For this review, take the finished solid that the model builds, in its own axes (mm). A direction names the side the tool comes from. Give positions to 0.01 mm unless a question says otherwise; leave off trailing zeros. Order: outer loops, then holes, each group sorted by start corner. A loop starts at its lowest first (then second) coordinate and runs counter-clockwise, first axis right, second up. Notation, with made-up numbers: (4, 35) - (32, 35) arc R11 ccw to (32, 42) - close; hole circle Ø6 at (27, 61). An arc over 180 degrees is marked (long way). Use a Markdown table: item, result. Add a question column.
1) We need section C-C on z = 32. Write out the cut boundary in (x, y).
2) Wall thickness on L1, parallel to Z at x = 15.5, y = -8.5; L2, parallel to Y at x = -6, z = 14.5; L3, parallel to Z at x = -15.5, y = -6.25: over which ranges is each line inside the solid? List them lowest first.
3) Machinability: for faces 5 (the face through (-17, -9, 10)), 6 (the face through (17, 0, 35)), 7 (the face through (0, -17, 5)), which of the approach directions +Z, -Z, +X, -X, +Y, -Y give a long, thin tool a straight path to every point of the face, cutting with its end or side? Answer none if there is none.
4) We need section D-D on y = -7.5. Write out the cut boundary in (x, z).
5) Mouldability with a two-part tool opening along Z and no side actions: class faces 1 (the face through (17, -9, 10)), 2 (the face through (20, -16, 20)), 3 (the face through (0, -16, 10)), 4 (the face through (0, -16, 40)) as released by +Z, released by -Z, zero draft, split by the parting line, or undercut.
6) We need section A-A on y = -4. Write out the cut boundary in (x, z).
7) We need section B-B on x = 0. Write out the cut boundary in (y, z).
8) Clearance check with flat-ended pins moving along their axes: P1, Ø3, axis at x = 0, z = 29, coming from the +Y side; P2, Ø1, axis at x = 14, z = 28.5, coming from the +Y side; P3, Ø0.6, axis at x = -1.5, y = -15.5, coming from the -Z side. State where each tip first meets the part, or that it passes through.
```python
from build123d import *

# Parameters (mm, degrees)
SKETCH1_W           = 40
SKETCH1_H           = 45
BOSS_EXTRUDE1_DEPTH = 40
SKETCH2_R           = 17
CUT_EXTRUDE1_DEPTH  = 10
SKETCH3_R           = 14
CUT_EXTRUDE2_DEPTH  = 10
SKETCH4_W           = 40
SKETCH4_H           = 22.5
CUT_EXTRUDE3_DEPTH  = 41
SKETCH5_W           = 40
SKETCH5_H           = 20
CUT_EXTRUDE4_DEPTH  = 15


with BuildPart() as part:
    # Sketch1 → Boss-Extrude1 (new body)
    with BuildSketch(Plane.XY):
        Rectangle(SKETCH1_W, SKETCH1_H)
    extrude(amount=BOSS_EXTRUDE1_DEPTH)

    # Sketch2 → Cut-Extrude1 (cut)
    with BuildSketch(Plane(origin=(0, 0, 0), x_dir=(-1, 0, 0), z_dir=(0, 0, -1))):
        Circle(SKETCH2_R)
    extrude(amount=-CUT_EXTRUDE1_DEPTH, mode=Mode.SUBTRACT)

    # Sketch3 → Cut-Extrude2 (cut)
    with BuildSketch(Plane.XY.offset(40)):
        Circle(SKETCH3_R)
    extrude(amount=-CUT_EXTRUDE2_DEPTH, mode=Mode.SUBTRACT)

    # Sketch4 → Cut-Extrude3 (cut, through all)
    with BuildSketch(Plane.XY.offset(40)):
        with Locations((0, 11.25)):
            Rectangle(SKETCH4_W, SKETCH4_H)
    extrude(amount=-CUT_EXTRUDE3_DEPTH, mode=Mode.SUBTRACT)

    # Sketch5 → Cut-Extrude4 (cut)
    with BuildSketch(Plane(origin=(0, 0, 0), x_dir=(1, 0, 0), z_dir=(0, 1, 0))):
        with Locations((0, -20)):
            Rectangle(SKETCH5_W, SKETCH5_H)
    extrude(amount=-CUT_EXTRUDE4_DEPTH, mode=Mode.SUBTRACT)


solid = part.part
```
Checked values:
| question | item | result |
|---|---|---|
| 1 | outline | (-20, -22.5) - (20, -22.5) - (20, 0) - (14, 0) arc R14 cw to (-14, 0) - (-20, 0) - close |
| 2 | L1 | 0 to 10, 30 to 40 |
| 2 | L2 | -22.5 to -15 |
| 2 | L3 | 30 to 40 |
| 3 | face 5 | +X, -X, +Y |
| 3 | face 6 | +Z, -Z, +X, -X, +Y |
| 3 | face 7 | -Z, +Y |
| 4 | outline | (-20, 0) - (-15.26, 0) - (-15.26, 10) - (-20, 10) - close; (-20, 30) - (-11.82, 30) - (-11.82, 40) - (-20, 40) - close; (11.82, 30) - (20, 30) - (20, 40) - (11.82, 40) - close; (15.26, 0) - (20, 0) - (20, 10) - (15.26, 10) - close |
| 5 | face 1 | undercut |
| 5 | face 2 | zero draft |
| 5 | face 3 | released by -Z |
| 5 | face 4 | released by +Z |
| 6 | outline | (-20, 0) - (-16.52, 0) - (-16.52, 10) - (-20, 10) - close; (-20, 30) - (-13.42, 30) - (-13.42, 40) - (-20, 40) - close; (13.42, 30) - (20, 30) - (20, 40) - (13.42, 40) - close; (16.52, 0) - (20, 0) - (20, 10) - (16.52, 10) - close |
| 7 | outline | (-22.5, 0) - (-17, 0) - (-17, 10) - (-15, 10) - (-15, 30) - (-14, 30) - (-14, 40) - (-22.5, 40) - close |
| 8 | P1 | y = -13.96 |
| 8 | P2 | y = -15 |
| 8 | P3 | z = 10 |
